The figure shows three views and two pictorial views of one solid part (mm, origin at its lowest corner). Answer the questions. Round coordinates to 2 decimals unless told otherwise and drop trailing zeros. Write each loop counter-clockwise with the first axis right and the second up, starting at its lowest first coordinate (ties: lowest second). Pieces come first, ordered by that corner, then holes.
Item 1: Find section C-C on z = 3. Give the vertices of the cut face in (x, y).
Item 2: Find section D-D on x = 200. Give the vertices of the cut face in (y, z), then the cut area to 3 significant figures.
Item 3: Find section B-B on x = 109.5. Give the vertices of the cut face in (y, z).
Item 4: Find section A-A on y = 45. Give the vertices of the cut face in (x, z).
Item 5: This flat-tipped pin is pushed along its axis until it touches: pin 1 (5 mm diameter, centred on x = 192, z = 4.5, fed in from -Y). Where does it stop, or does it pass through?
Item 6: For a pull along X with two mould halves and no side action, classify the marked faces 1 and 2 as +X half, -X half, draft (parallel to the pull), parting line (faces both ways), or undercut.
Item 7: Find the intervals of material crossed by probe 1 along X at (y, z) = (23.5, 4.25); probe 2 along Y at (x, z) = (200, 6.5); probe 3 along Y at (x, z) = (156, 3), in increasing order.
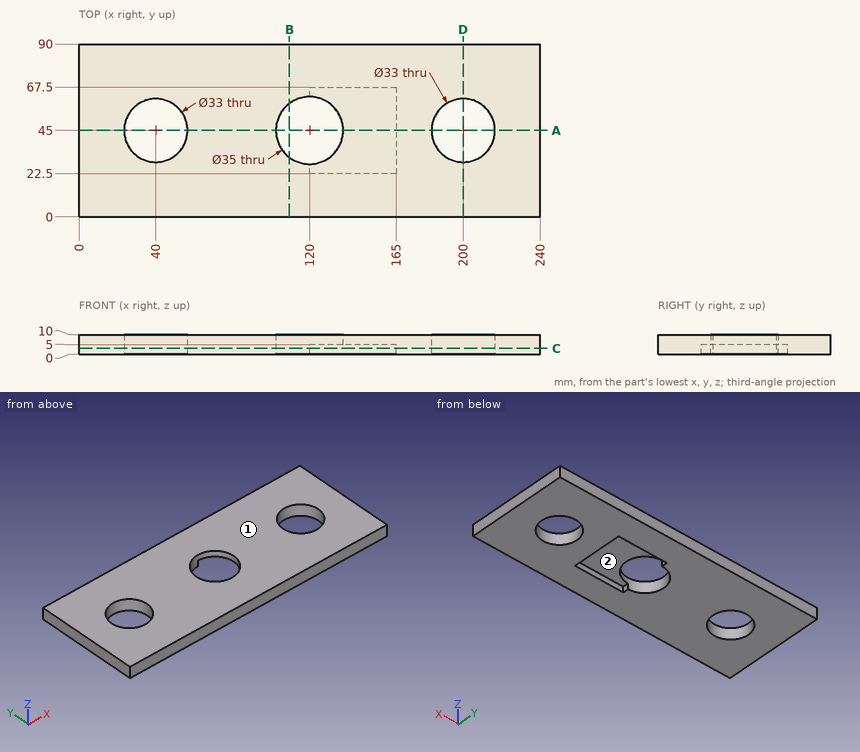
Check values:
1. outline: (0, 0) - (240, 0) - (240, 90) - (0, 90) - close; hole circle Ø33 at (40, 45); hole (120, 22.5) - (165, 22.5) - (165, 67.5) - (120, 67.5) - (120, 62.5) arc R17.5 ccw to (120, 27.5) - close; hole circle Ø33 at (200, 45)
2. outline: (0, 0) - (28.5, 0) - (28.5, 10) - (0, 10) - close; (61.5, 0) - (90, 0) - (90, 10) - (61.5, 10) - close
2. area: 570 mm2
3. outline: (0, 0) - (31, 0) - (31, 10) - (0, 10) - close; (59, 0) - (90, 0) - (90, 10) - (59, 10) - close
4. outline: (0, 0) - (23.5, 0) - (23.5, 10) - (0, 10) - close; (56.5, 0) - (102.5, 0) - (102.5, 10) - (56.5, 10) - close; (137.5, 5) - (165, 5) - (165, 0) - (183.5, 0) - (183.5, 10) - (137.5, 10) - close; (216.5, 0) - (240, 0) - (240, 10) - (216.5, 10) - close
5. pin 1: stops at y = 0
6. face 1: draft
6. face 2: undercut
7. probe 1: x = 0 to 120, 165 to 240
7. probe 2: y = 0 to 28.5, 61.5 to 90
7. probe 3: y = 0 to 22.5, 67.5 to 90
